Check sheet for the modelled part. Datum: model origin and axes. Units: mm. A direction names the side the tool comes from. Coordinates: 2 decimals unless noted, no trailing zeros. Order: outer loops, then holes, each group sorted by start corner. A loop starts at its lowest first (then second) coordinate and runs counter-clockwise, first axis right, second up.
1. Draft check along Y on faces 1 (the flat face through (20, 28.5, 5)), 2 (the flat face through (20, 14, 0)), 3 (the flat face through (22, 2, 5)). Enter one of: released by +Y, released by -Y, zero draft, split by the parting line, or undercut.
2. Cross-section at B-B (x = 31). Enter the section's corners in (y, z), then the cut area to 3 significant figures.
3. Gauge pin test, flat ends, axial feed: pin 1 Ø3 at (x, y) = (27, 10.5) entering from +Z; pin 2 Ø2.5 at (y, z) = (12, 7) entering from +X; pin 3 Ø0.6 at (x, y) = (6, 27.5) entering from +Z. Record the tip position at first contact, or that the pin passes through.
4. Cross-section at A-A (z = 7.5). Enter the section's corners in (x, y), then the cut area to 3 significant figures.
5. Cross-section at C-C (y = 4). Enter the section's corners in (x, z), then the cut area to 3 significant figures.
6. Cross-section at D-D (y = 11.25). Enter the section's corners in (x, z).
7. Set-up check for faces 4 (the flat face through (21, 14, 4)), 5 (the flat face through (9, 28, 7)), 6 (the flat face through (29, 28, 10)): record each of +Z, -Z, +X, -X, +Y, -Y from which the full face is reachable in a straight line by a thin tool's end or side.
8. Thickness scan on line 1 (Y direction, x = 19.5, z = 5); line 2 (X direction, y = 18.25, z = 9.25); line 3 (Z direction, x = 39.5, y = 20.5). Record the ranges inside material, lowest first.
```python
from build123d import *

# Parameters (mm, degrees)
F1_DEPTH = 1
F0_W     = 39
F0_H     = 4
F0_H_2   = 16.5
F2_DEPTH = 4
F0_W_2   = 15
F0_H_3   = 2
F3_DEPTH = 7
F0_W_3   = 24
F4_DEPTH = 10


# Not quite as in the source:
# - a feature names something its author has since deleted; it is built from what else it names


with BuildPart() as f1:
    # F0 (on Top) → F1 (new body)
    with BuildSketch(Plane.XY):
        Polygon((17, 26.5), (2, 26.5), (2, 22.5), (41, 22.5), (41, 26.5), align=None)
    extrude(amount=F1_DEPTH)



with BuildPart() as f1b:
    # F0 (on Top) → F1, piece 2 (new body)
    with BuildSketch(Plane.XY):
        with Locations((21.5, 4)):
            Rectangle(F0_W, F0_H)
    extrude(amount=F1_DEPTH)


with BuildPart() as f1_1:
    add(f1.part)

    add(f1b.part)  # F2 merges F1b
    # F0 (on Top) → F2 (join)
    with BuildSketch(Plane.XY):
        with Locations((21.5, 14.25)):
            Rectangle(F0_W, F0_H_2)
    extrude(amount=F2_DEPTH)

    # F0 (on Top) → F3 (join)
    with BuildSketch(Plane.XY):
        with Locations((9.5, 27.5)):
            Rectangle(F0_W_2, F0_H_3)
    extrude(amount=F3_DEPTH)

    # F0 (on Top) → F4 (join)
    with BuildSketch(Plane.XY):
        with Locations((29, 27.5)):
            Rectangle(F0_W_3, F0_H_3)
        Polygon((2, 22.5), (2, 26.5), (2, 28.5), (0, 28.5), (0, 2), (2, 2), (2, 6), align=None)
        Polygon((41, 2), (2, 2), (0, 2), (0, 0), (41, 0), align=None)
    extrude(amount=F4_DEPTH)


solid = f1_1.part
```
Data:
1. face 1: released by +Y
1. face 2: zero draft
1. face 3: undercut
2. outline: (0, 0) - (28.5, 0) - (28.5, 10) - (26.5, 10) - (26.5, 1) - (22.5, 1) - (22.5, 4) - (6, 4) - (6, 1) - (2, 1) - (2, 10) - (0, 10) - close
2. area: 114 mm2
3. pin 1: stops at z = 4
3. pin 2: stops at x = 2
3. pin 3: stops at z = 7
4. outline: (0, 0) - (41, 0) - (41, 2) - (2, 2) - (2, 28.5) - (0, 28.5) - close; (17, 26.5) - (41, 26.5) - (41, 28.5) - (17, 28.5) - close
4. area: 183 mm2
5. outline: (0, 0) - (41, 0) - (41, 1) - (2, 1) - (2, 10) - (0, 10) - close
5. area: 59.0 mm2
6. outline: (0, 0) - (41, 0) - (41, 4) - (2, 4) - (2, 10) - (0, 10) - close
7. face 4: +Z, +X
7. face 5: +Z, +Y
7. face 6: +Z, +X, -X, +Y, -Y
8. line 1: y = 0 to 2, 26.5 to 28.5
8. line 2: x = 0 to 2
8. line 3: z = 0 to 4
